from build123d import *

# Parameters (mm, degrees)
SKETCH1_RX          = 140
SKETCH1_RY          = 90
BOSS_EXTRUDE1_DEPTH = 15
SKETCH2_W           = 60
SKETCH2_H           = 30
BOSS_EXTRUDE2_DEPTH = 35
SKETCH3_W           = 525
SKETCH3_H           = 50
BOSS_EXTRUDE3_DEPTH = 350


with BuildPart() as part:
    # Sketch1 → Boss-Extrude1 (new body)
    with BuildSketch(Plane(origin=(0, 0, 0), x_dir=(1, 0, 0), z_dir=(0, 1, 0))):
        with Locations((0, 0)):
            Ellipse(SKETCH1_RX, SKETCH1_RY)
    extrude(amount=BOSS_EXTRUDE1_DEPTH)

    # Sketch2 → Boss-Extrude2 (add)
    with BuildSketch(Plane(origin=(0, 15, 0), x_dir=(1, 0, 0), z_dir=(0, 1, 0))):
        Rectangle(SKETCH2_W, SKETCH2_H)
    extrude(amount=BOSS_EXTRUDE2_DEPTH)

    # Sketch3 → Boss-Extrude3 (add)
    with BuildSketch(Plane(origin=(0, 50, 0), x_dir=(1, 0, 0), z_dir=(0, 1, 0))):
        Rectangle(SKETCH3_W, SKETCH3_H)
    extrude(amount=BOSS_EXTRUDE3_DEPTH)


solid = part.part
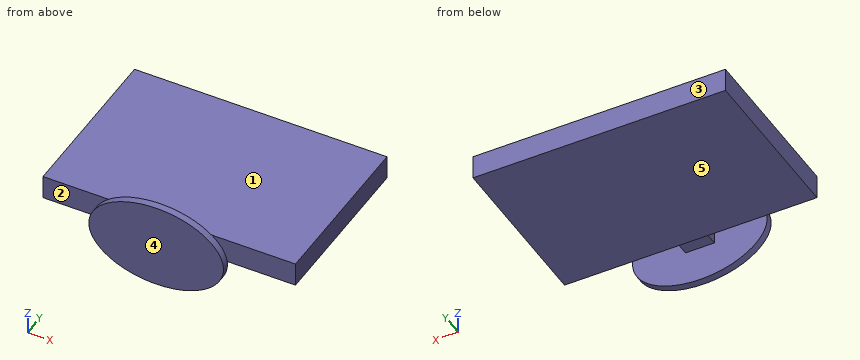
The model under review builds one solid part; all positions refer to its coordinate system, in mm. Face numbers are marked on the shaded views. A direction names the side the tool comes from. Give positions to 0.01 mm unless a question says otherwise; leave off trailing zeros. Loops run counter-clockwise (first coordinate to the right, second up) from the corner with the lowest first, then second, coordinate; pieces in that order, holes last. Notation, with made-up numbers: (87.5, -40) -> (95.5, -40) arc R16 ccw to (95.5, -10) -> close; hole circle Ø10 at (1, -37). An arc over 180 degrees is marked (long way). Put each result on its own line as item: value. Start each with the question number.
1. We need section A-A on x = 228.5. State the section outline as (y, z) points.
2. For the marked faces 4 and 5, list the 3-axis set-ups (+Z, -Z, +X, -X, +Y, -Y) from which the entire face can be reached by the end or side of a thin tool; tool diameter is ignored.
3. Mouldability with a two-part tool opening along Y and no side actions: class the marked faces 1, 2 and 3 as released by +Y, released by -Y, zero draft, split by the parting line, or undercut.
4. Wall thickness on probe 1 along Y at (x, z) = (51, 17.5); probe 2 along Y at (x, z) = (-118, 45); probe 3 along Z at (x, y) = (-120, 356.5): over which ranges is each line inside the solid? List them lowest first.
5. We need section B-B on y = 339.5. State the section outline as (x, z) points.
6. Clearance check with flat-ended pins moving along their axes: P1, Ø24, axis at y = 28, z = 7, coming from the -X side; P2, Ø9, axis at y = 24.5, z = 1, coming from the +X side; P3, Ø3, axis at x = -195.5, y = 186.5, coming from the -Z side. State where each tip first meets the part, or that it passes through.
Determined:
1. outline: (50, -25) -> (400, -25) -> (400, 25) -> (50, 25) -> close
2. face 4: +Z, -Z, +X, -X, -Y
2. face 5: -Z, +X, -X, +Y
3. face 1: zero draft
3. face 2: undercut
3. face 3: released by +Y
4. probe 1: 0 to 15, 50 to 400
4. probe 2: 0 to 15
4. probe 3: -25 to 25
5. outline: (-262.5, -25) -> (262.5, -25) -> (262.5, 25) -> (-262.5, 25) -> close
6. P1: x = -30
6. P2: x = 30
6. P3: z = -25
